Answer from the drawing. Dimensions are ordinates in mm from the lowest x, y and z of the part. Coordinates: 2 decimals unless noted, no trailing zeros. Write each loop counter-clockwise with the first axis right and the second up, starting at its lowest first coordinate (ties: lowest second). Pieces come first, ordered by that corner, then holes.
(1) Determine the mould class of the marked faces 1, 2 and 3 for opening direction X: pulls with the +X half, pulls with the -X half, needs draft (parallel to the pull), parting line crosses it, or undercut.
(2) Given pin 1 (4 mm diameter, centred on x = 8.86, y = 31.14, fed in from +Z); pin 2 (6 mm diameter, centred on x = 8.86, y = 8.86, fed in from +Z), each flat-ended and moving along its own axis, determine where each tip first touches the part or whether it passes through.
(3) The part is cut by section D-D, the plane z = 7.5. Determine the outline of the cut face in (x, y).
(4) The part is cut by section C-C, the plane z = 5.25. Determine the outline of the cut face in (x, y), and give its area (3 significant figures).
(5) Straight lines are drawn through the part: line 1 along Y through (x, z) = (20, 4.25); line 2 along Y through (x, z) = (8, 6.5); line 3 along Y through (x, z) = (30.5, 4). For each, find the intervals that lie inside material, in ascending order.
(6) The part is cut by section B-B, the plane x = 20. Determine the outline of the cut face in (y, z).
(7) The part is cut by section A-A, the plane y = 20. Determine the outline of the cut face in (x, z).
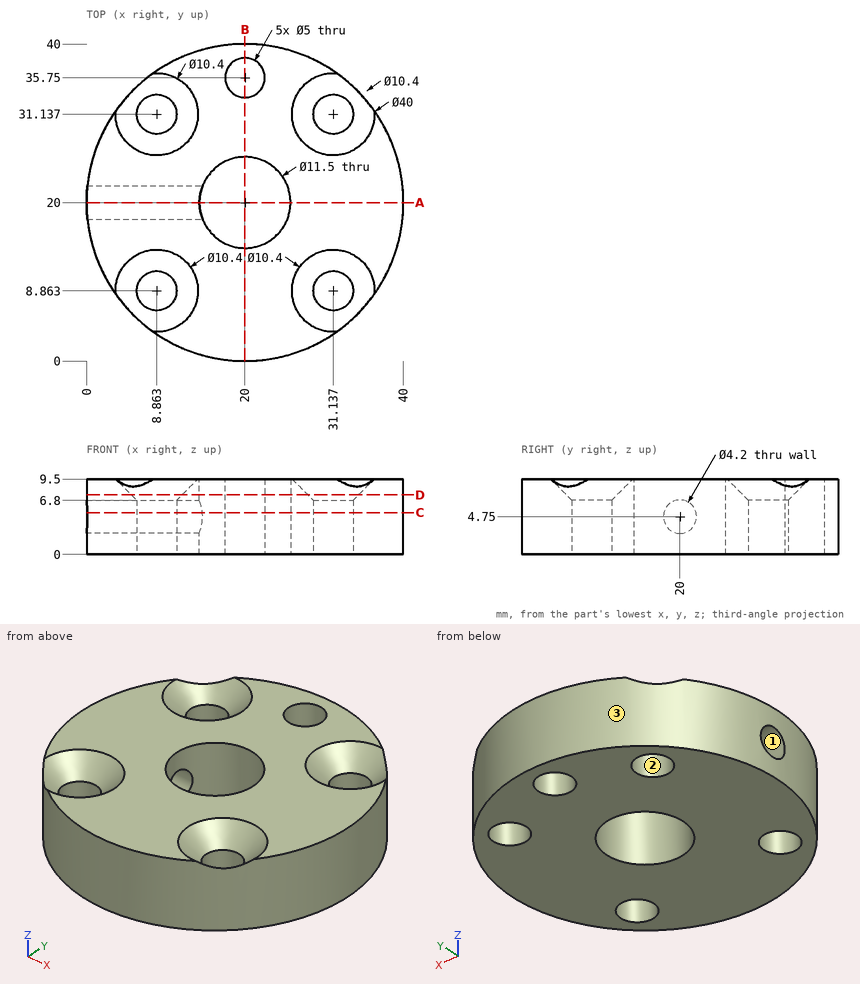
Computed:
1. face 1: needs draft
1. face 2: undercut
1. face 3: parting line crosses it
2. pin 1: passes through
2. pin 2: stops at z = 7.3
3. outline: circle Ø40 at (20, 20); hole circle Ø6.4 at (8.86, 8.86); hole circle Ø6.4 at (8.86, 31.14); hole circle Ø11.5 at (20, 20); hole circle Ø5 at (20, 35.75); hole circle Ø6.4 at (31.14, 8.86); hole circle Ø6.4 at (31.14, 31.14)
4. outline: (0.1, 17.96) arc R20 ccw (long way) to (0.1, 22.04) - (14.62, 22.04) arc R5.75 cw (long way) to (14.62, 17.96) - close; hole circle Ø5 at (8.86, 8.86); hole circle Ø5 at (8.86, 31.14); hole circle Ø5 at (20, 35.75); hole circle Ø5 at (31.14, 8.86); hole circle Ø5 at (31.14, 31.14)
4. area: 996 mm2
5. line 1: y = 0 to 14.25, 25.75 to 33.25, 38.25 to 40
5. line 2: y = 4 to 6.52, 11.21 to 18.84, 21.16 to 28.79, 33.48 to 36
5. line 3: y = 2.98 to 6.45, 11.28 to 28.72, 33.55 to 37.02
6. outline: (0, 0) - (14.25, 0) - (14.25, 9.5) - (0, 9.5) - close; (25.75, 0) - (33.25, 0) - (33.25, 9.5) - (25.75, 9.5) - close; (38.25, 0) - (40, 0) - (40, 9.5) - (38.25, 9.5) - close
7. outline: (0, 0) - (14.25, 0) - (14.25, 2.65) - (0, 2.65) - close; (0, 6.85) - (14.25, 6.85) - (14.25, 9.5) - (0, 9.5) - close; (25.75, 0) - (40, 0) - (40, 9.5) - (25.75, 9.5) - close
